from build123d import *

# Parameters (mm, degrees)
SKETCH1_W           = 85
SKETCH1_H           = 70
BOSS_EXTRUDE1_DEPTH = 75
SKETCH2_W           = 75
SKETCH2_H           = 60
CUT_EXTRUDE1_DEPTH  = 70
SKETCH3_W           = 20
SKETCH3_H           = 20
BOSS_EXTRUDE2_DEPTH = 25


with BuildPart() as part:
    # Sketch1 → Boss-Extrude1 (new body)
    with BuildSketch(Plane(origin=(0, 0, 0), x_dir=(1, 0, 0), z_dir=(0, 1, 0))):
        with Locations((42.5, 35)):
            Rectangle(SKETCH1_W, SKETCH1_H)
    extrude(amount=BOSS_EXTRUDE1_DEPTH)

    # Sketch2 → Cut-Extrude1 (cut)
    with BuildSketch(Plane(origin=(0, 75, 0), x_dir=(1, 0, 0), z_dir=(0, 1, 0))):
        with Locations((42.5, 35)):
            Rectangle(SKETCH2_W, SKETCH2_H)
    extrude(amount=-CUT_EXTRUDE1_DEPTH, mode=Mode.SUBTRACT)

    # Sketch3 → Boss-Extrude2 (add)
    with BuildSketch(Plane(origin=(0, 5, 0), x_dir=(1, 0, 0), z_dir=(0, 1, 0))):
        with Locations((65, 32.492591032)):
            Rectangle(SKETCH3_W, SKETCH3_H)
    extrude(amount=BOSS_EXTRUDE2_DEPTH)


solid = part.part
Part model, mm, in its own coordinate system. A direction names the side the tool comes from. Coordinates: 2 decimals unless noted, no trailing zeros. Loops run counter-clockwise (first coordinate to the right, second up) from the corner with the lowest first, then second, coordinate; pieces in that order, holes last. Notation, with made-up numbers: (37.5, 8.25) - (55.5, 8.25) arc R12 cw to (55.5, 19.25) - close; hole circle Ø4 at (70.25, 32). An arc over 180 degrees is marked (long way). Write each question's results on one line, items separated by ' | '. Start each with the question number.
Q1. Drop flat-ended pins along their axis: pin 1 Ø22 at (x, z) = (68.5, -34.5) entering from +Y; pin 2 Ø6 at (x, z) = (31, -55) entering from +Y. Give the stop position or say it passes through.
Q2. Slice it at B-B on z = -33. Give the cut face in (x, y).
Q3. Two-plate mould, pull along Z, no slides. Class faces 1 (the flat face through (42, 75, -66)), 2 (the flat face through (42, 37, 0)), 3 (the flat face through (55, 17, -32)): +Z half, -Z half, draft (parallel to the pull), parting line (faces both ways), or undercut.
Q4. Slice it at A-A on y = 18.5. Give the cut face in (x, z).
Q5. Which spindle directions (+Z, -Z, +X, -X, +Y, -Y) get a long thin tool onto all of the face, cutting with end or side? Do faces 4 (the flat face through (85, 37, -35)), 5 (the flat face through (42, 40, -5)). Say none if no direction does.
Q6. Probe line 1 along X through (y, z) = (25, -31); line 2 along Z through (x, y) = (56, 20); line 3 along X through (y, z) = (33.5, -6). List the from-to ranges inside material, lowest first.
Q7. Slice it at C-C on x = 58.5. Give the cut face in (y, z).
Q8. Slice it at D-D on y = 66. Give the cut face in (x, z), and give its area (3 significant figures).
Answer:
1) pin 1: stops at y = 30 | pin 2: stops at y = 5
2) outline: (0, 0) - (85, 0) - (85, 75) - (80, 75) - (80, 5) - (75, 5) - (75, 30) - (55, 30) - (55, 5) - (5, 5) - (5, 75) - (0, 75) - close
3) face 1: draft | face 2: +Z half | face 3: undercut
4) outline: (0, -70) - (85, -70) - (85, 0) - (0, 0) - close; (55, -42.49) - (75, -42.49) - (75, -22.49) - (55, -22.49) - close; hole (5, -65) - (80, -65) - (80, -5) - (5, -5) - close
5) face 4: +Z, -Z, +X, +Y, -Y | face 5: +Y
6) line 1: x = 0 to 5, 55 to 75, 80 to 85 | line 2: z = -70 to -65, -42.49 to -22.49, -5 to 0 | line 3: x = 0 to 5, 80 to 85
7) outline: (0, -70) - (75, -70) - (75, -65) - (5, -65) - (5, -42.49) - (30, -42.49) - (30, -22.49) - (5, -22.49) - (5, -5) - (75, -5) - (75, 0) - (0, 0) - close
8) outline: (0, -70) - (85, -70) - (85, 0) - (0, 0) - close; hole (5, -65) - (80, -65) - (80, -5) - (5, -5) - close | area: 1,450 mm2
